from build123d import *

# Parameters (mm, degrees)
F0_W     = 127
F0_H     = 101.6
F0_W_2   = 101.6
F0_H_2   = 76.2
F1_DEPTH = 101.6
F2_W     = 54.790769
F2_H     = 39.199134
F3_DEPTH = 152.4
F4_R     = 12.7
F5_DEPTH = 203.2


with BuildPart() as f1:
    # F0 (on Top) → F1 (new body)
    with BuildSketch(Plane.XY):
        with Locations((29.390769, 2.499611)):
            Rectangle(F0_W, F0_H)
        with Locations((29.390769, 2.499611)):
            Rectangle(F0_W_2, F0_H_2, mode=Mode.SUBTRACT)
    extrude(amount=F1_DEPTH)

    # F2 (on face) → F3 (cut)
    with BuildSketch(Plane.XZ.offset(48.300389)):
        with Locations((27.395384, 82.000433)):
            Rectangle(F2_W, F2_H)
    extrude(amount=-F3_DEPTH, mode=Mode.SUBTRACT)

    # F4 (on face) → F5 (cut)
    with BuildSketch(Plane(origin=(-34.109231, 0, 0), x_dir=(0, -1, 0), z_dir=(-1, 0, 0))):
        with Locations((-2.499611, 50.8)):
            Circle(F4_R)
    extrude(amount=-F5_DEPTH, mode=Mode.SUBTRACT)


solid = f1.part
The listing builds one solid part. Answer for the finished solid, in the listing's coordinates (mm). A direction names the side the tool comes from. Give positions to 0.01 mm unless a question says otherwise; leave off trailing zeros. Write each loop counter-clockwise with the first axis right and the second up, starting at its lowest first coordinate (ties: lowest second). Pieces come first, ordered by that corner, then holes. Notation, with made-up numbers: (83.25, -22) - (93.25, -22) arc R16 cw to (93.25, -8) - close; hole circle Ø11 at (-21, 45). An arc over 180 degrees is marked (long way). Use a Markdown table: item, result.
1. Section A-A on x = -11.5 is taken. Write down the section's boundary in (y, z).
Values follow:
| item | result |
|---|---|
| outline | (-48.3, 0) - (-35.6, 0) - (-35.6, 101.6) - (-48.3, 101.6) - close; (40.6, 0) - (53.3, 0) - (53.3, 101.6) - (40.6, 101.6) - close |
2. Section B-B on z = 95.5 is taken. Write down the section's boundary in (x, y).
Values follow:
| item | result |
|---|---|
| outline | (-34.11, -48.3) - (0, -48.3) - (0, -35.6) - (-21.41, -35.6) - (-21.41, 40.6) - (0, 40.6) - (0, 53.3) - (-34.11, 53.3) - close; (54.79, -48.3) - (92.89, -48.3) - (92.89, 53.3) - (54.79, 53.3) - (54.79, 40.6) - (80.19, 40.6) - (80.19, -35.6) - (54.79, -35.6) - close |
3. Section C-C on y = -31.5 is taken. Write down the section's boundary in (x, z).
Values follow:
| item | result |
|---|---|
| outline | (-34.11, 0) - (-21.41, 0) - (-21.41, 101.6) - (-34.11, 101.6) - close; (80.19, 0) - (92.89, 0) - (92.89, 101.6) - (80.19, 101.6) - close |
4. This flat-tipped pin is pushed along its axis until it touches: P1, Ø14, axis at x = 17, y = 48, coming from the +Z side. Where does it stop, or does it pass through?
Values follow:
| item | result |
|---|---|
| P1 | stops at z = 62.4 |
5. Section D-D on z = 32 is taken. Write down the section's boundary in (x, y), plus the area to 3 significant figures.
Values follow:
| item | result |
|---|---|
| outline | (-34.11, -48.3) - (92.89, -48.3) - (92.89, 53.3) - (-34.11, 53.3) - close; hole (-21.41, -35.6) - (80.19, -35.6) - (80.19, 40.6) - (-21.41, 40.6) - close |
| area | 5,160 mm² |
6. A tool of negligible diameter and unlimited length cuts with its end or side. For faces 5 (the flat face through (54.791, -42, 82)), 6 (the flat face through (-21.409, -7, 61)), 7 (the flat face through (-25, 3, 101.6)), from which of +Z, -Z, +X, -X, +Y, -Y can it reach the whole face along a straight path? Write none if from no direction.
Values follow:
| item | result |
|---|---|
| face 5 | +Z, +Y, -Y |
| face 6 | +Z, -Z |
| face 7 | +Z, +X, -X, +Y, -Y |
7. Find the intervals of material crossed by probe 1 along Y at (x, z) = (-24, 50); probe 2 along X at (y, z) = (-13, 49.5); probe 3 along Y at (x, z) = (51, 30.5), in increasing order. Write a range as from..to.
Values follow:
| item | result |
|---|---|
| probe 1 | y = -48.3..-10.18, 15.17..53.3 |
| probe 2 | x = -34.11..-21.41, 80.19..92.89 |
| probe 3 | y = -48.3..-35.6, 40.6..53.3 |
8. For a pull along Z with two mould halves and no side action, classify faces 1 (the flat face through (29, -42, 0)), 2 (the cylindrical face through (86.452, -3.361, 39.533)), 3 (the flat face through (82, 3, 101.6)), 4 (the flat face through (92.891, -10, 61)) as released by +Z, released by -Z, zero draft, split by the parting line, or undercut.
Values follow:
| item | result |
|---|---|
| face 1 | released by -Z |
| face 2 | undercut |
| face 3 | released by +Z |
| face 4 | zero draft |
